Verification items for the finished model (mm, model axes). Face numbers are marked on the shaded views. Coordinates: 2 decimals unless noted, no trailing zeros. Order: outer loops, then holes, each group sorted by start corner. A loop starts at its lowest first (then second) coordinate and runs counter-clockwise, first axis right, second up. Notation, with made-up numbers: (-7, 79.25) -> (14, 79.25) arc R20 ccw to (14, 101.25) -> close; hole circle Ø4 at (-1, 17.5). An arc over 180 degrees is marked (long way). Use CSV: the item, a comma, the result in double quotes. Start each with the question number.
1) Sectioned sample at C-C on y = 4.85. Record the boundary of the cut face in (x, z), then the cut area to 3 significant figures.
2) Scan lines: line 1 along X through (y, z) = (3.3, 0); line 2 along Z through (x, y) = (0, 1.45); line 3 along X through (y, z) = (2.1, -0.25). Record each from-to range of solid material in increasing order.
3) Release check for a two-part mould opening along X. For the marked faces 1, 2, 3 and 4 record: released by +X, released by -X, zero draft, split by the parting line, or undercut.
4) Sectioned sample at A-A on x = 0. Record the boundary of the cut face in (y, z), then the cut area to 3 significant figures.
5) Sectioned sample at B-B on z = 0. Record the boundary of the cut face in (x, y), then the cut area to 3 significant figures.
from build123d import *

# Parameters (mm, degrees)
SKETCH1_W           = 40.005
SKETCH1_H           = 9.0424
BOSS_EXTRUDE1_DEPTH = 5.334
SKETCH2_R           = 2.159
CUT_EXTRUDE1_DEPTH  = 6.334


with BuildPart() as part:
    # Sketch1 → Boss-Extrude1 (new body)
    with BuildSketch(Plane(origin=(0, 0, 0), x_dir=(1, 0, 0), z_dir=(0, 1, 0))):
        Rectangle(SKETCH1_W, SKETCH1_H)
    extrude(amount=BOSS_EXTRUDE1_DEPTH)

    # Sketch2 → Cut-Extrude1 (cut, through all)
    with BuildSketch(Plane(origin=(0, 5.334, 0), x_dir=(1, 0, 0), z_dir=(0, 1, 0))):
        Circle(SKETCH2_R)
    extrude(amount=-CUT_EXTRUDE1_DEPTH, mode=Mode.SUBTRACT)


solid = part.part
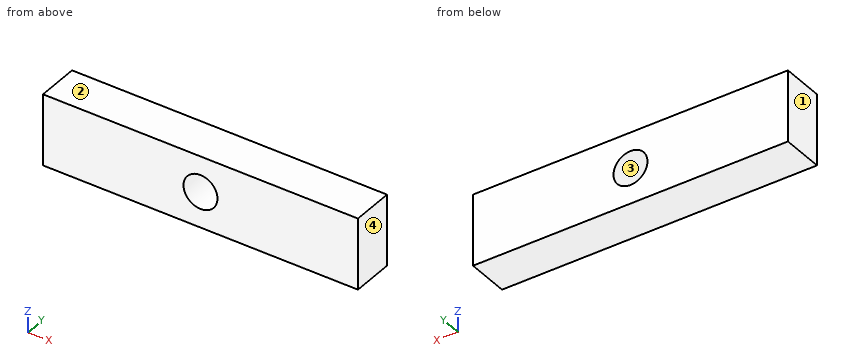
Answers follow:
1,outline,"(-20, -4.52) -> (20, -4.52) -> (20, 4.52) -> (-20, 4.52) -> close; hole circle Ø4.32 at (0, 0)"
1,area,"347 mm²"
2,line 1,"x = -20 to -2.16, 2.16 to 20"
2,line 2,"z = -4.52 to -2.16, 2.16 to 4.52"
2,line 3,"x = -20 to -2.14, 2.14 to 20"
3,face 1,"released by -X"
3,face 2,"zero draft"
3,face 3,"undercut"
3,face 4,"released by +X"
4,outline,"(0, -4.52) -> (5.33, -4.52) -> (5.33, -2.16) -> (0, -2.16) -> close; (0, 2.16) -> (5.33, 2.16) -> (5.33, 4.52) -> (0, 4.52) -> close"
4,area,"25.2 mm²"
5,outline,"(-20, 0) -> (-2.16, 0) -> (-2.16, 5.33) -> (-20, 5.33) -> close; (2.16, 0) -> (20, 0) -> (20, 5.33) -> (2.16, 5.33) -> close"
5,area,"190 mm²"
